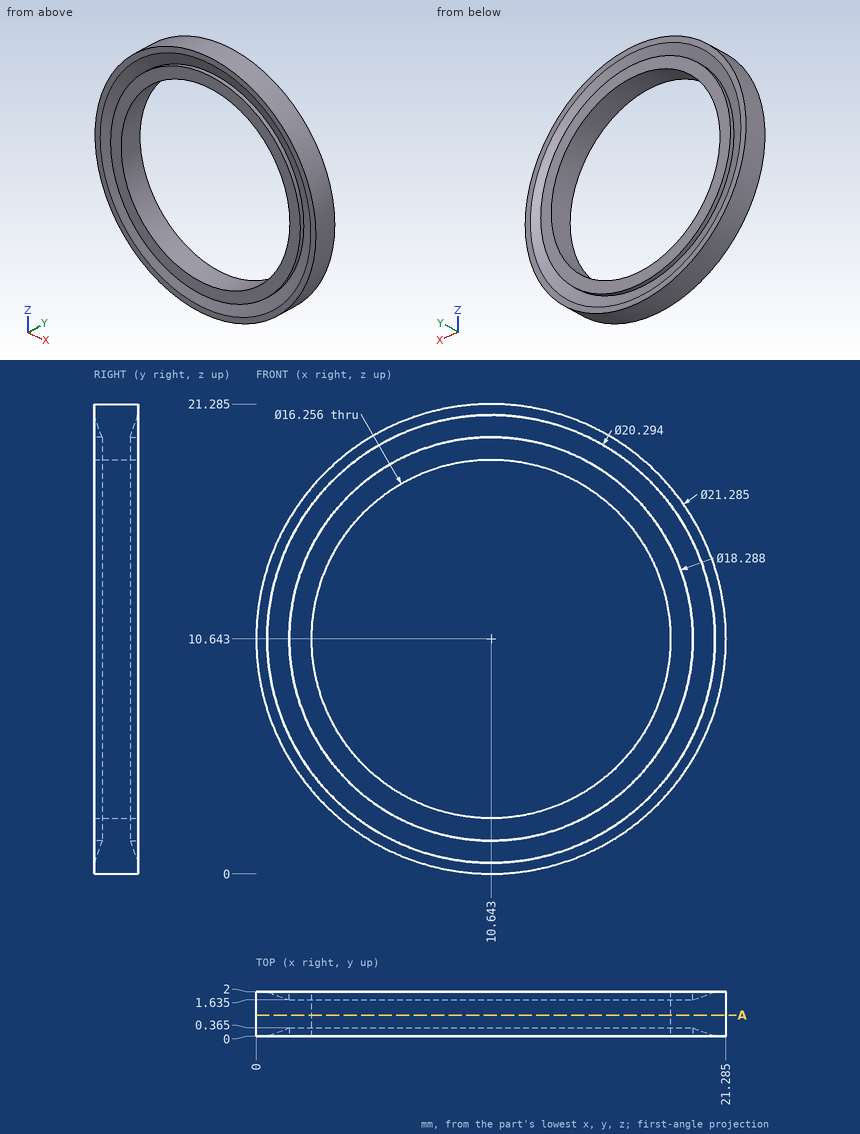
Input: dimensioned drawing with shaded views. Units: mm. Origin: part minimum x, y, z. Coordinates: 2 decimals unless noted, no trailing zeros. Order: outer loops, then holes, each group sorted by start corner. A loop starts at its lowest first (then second) coordinate and runs counter-clockwise, first axis right, second up. Notation, with made-up numbers: (75, 4.5) - (127, 4.5) arc R19 ccw to (127, 16.5) - close; hole circle Ø3 at (83.25, 70.25). An arc over 180 degrees is marked (long way). Return JSON: item names as keys, results as strings. Group by question number.
1. Material intervals for line 1 along Z through (x, y) = (16.5, 1) (1 decimal); line 2 along X through (y, z) = (0.75, 9); line 3 along Z through (x, y) = (17.75, 0.5) (1 decimal), sorted ascending. Write a range as [from, to].
2. Pin query (flat end, axial travel): pin 1 (5 mm diameter, centred on x = 18.5, z = 16.5, fed in from -Y); pin 2 (1 mm diameter, centred on x = 9, y = 1, fed in from +Z). Return the tip coordinate at first contact, or that it passes through.
3. Cut plane A-A (y = 0.95). Output: boundary loops of the cut face in (x, z) (1 decimal).
Resolved:
{
 "1": {"line 1": "z = [1.8, 5], [16.3, 19.5]", "line 2": "x = [0.13, 2.68], [18.6, 21.16]", "line 3": "z = [2.7, 6.7], [14.6, 18.6]"},
 "2": {"pin 1": "stops at y = 0", "pin 2": "stops at z = 21.22"},
 "3": {"outline": "circle Ø21.3 at (10.6, 10.6); hole circle Ø16.3 at (10.6, 10.6)"}
}
